Part model, mm, in its own coordinate system. Face numbers are marked on the shaded views. Give positions to 0.01 mm unless a question says otherwise; leave off trailing zeros. Order: outer loops, then holes, each group sorted by start corner. A loop starts at its lowest first (then second) coordinate and runs counter-clockwise, first axis right, second up. Notation, with made-up numbers: M 3,64 L 24,64 A21 ccw 24,76 Z; hole C 11,55 d2. An arc over 180 degrees is marked long. Return JSON: item names as keys, results as strings.
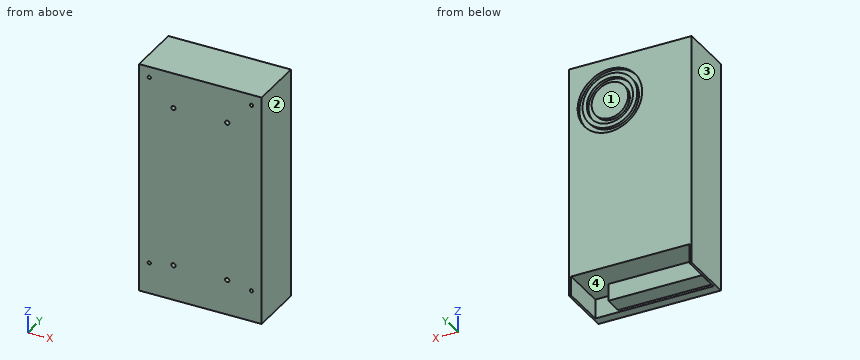
from build123d import *

# Parameters (mm, degrees)
SKETCH_2_W          = 114
SKETCH_2_H          = 216
EXTRUDE_2_DEPTH     = 51
SKETCH_3_R          = 1.5
SKETCH_3_R_2        = 2
CUT_EXTRUDE_1_DEPTH = 10
SKETCH_4_W          = 110
SKETCH_4_H          = 18
CUT_EXTRUDE_2_DEPTH = 42
SKETCH_5_W          = 87
SKETCH_5_H          = 16
EXTRUDE_3_DEPTH     = 17
SKETCH_6_R          = 30
SKETCH_6_R_2        = 25.436388115
CUT_EXTRUDE_4_DEPTH = 3
SKETCH_7_R          = 21.493717547
SKETCH_7_R_2        = 16.968980291
CUT_EXTRUDE_5_DEPTH = 3


with BuildPart() as part:
    # Эскиз2 → Бобышка-Вытянуть2 (new body)
    with BuildSketch(Plane(origin=(0, 0, 0), x_dir=(1, 0, 0), z_dir=(0, 1, 0))):
        with Locations((45.595035846, -62.514319432)):
            Rectangle(SKETCH_2_W, SKETCH_2_H)
    extrude(amount=EXTRUDE_2_DEPTH)

    # Эскиз3 → Вырез-Вытянуть1 (cut)
    with BuildSketch(Plane.XZ):
        with Locations(Location((-1.904964154, 160.514319432, 0), (0, 0, 270))):
            Circle(SKETCH_3_R)
        with Locations(Location((93.095035846, 160.514319432, 0), (0, 0, 270))):
            Circle(SKETCH_3_R)
        with Locations(Location((-1.904964154, -16.485680568, 0), (0, 0, 270))):
            Circle(SKETCH_3_R)
        with Locations(Location((93.095035846, -16.485680568, 0), (0, 0, 270))):
            Circle(SKETCH_3_R)
        with Locations(Location((20.595035846, 137.514319432, 0), (0, 0, 270))):
            Circle(SKETCH_3_R_2)
        with Locations(Location((70.595035846, 137.514319432, 0), (0, 0, 270))):
            Circle(SKETCH_3_R_2)
        with Locations(Location((20.595035846, -12.485680568, 0), (0, 0, 270))):
            Circle(SKETCH_3_R_2)
        with Locations(Location((70.595035846, -12.485680568, 0), (0, 0, 270))):
            Circle(SKETCH_3_R_2)
    extrude(amount=-CUT_EXTRUDE_1_DEPTH, mode=Mode.SUBTRACT)

    # Эскиз4 → Вырез-Вытянуть2 (cut)
    with BuildSketch(Plane(origin=(0, 51, 0), x_dir=(1, 0, 0), z_dir=(0, 1, 0))):
        with Locations((45.595035846, 36.485680568)):
            Rectangle(SKETCH_4_W, SKETCH_4_H)
    extrude(amount=-CUT_EXTRUDE_2_DEPTH, mode=Mode.SUBTRACT)

    # Эскиз5 → Бобышка-Вытянуть3 (add)
    with BuildSketch(Plane(origin=(0, 9, 0), x_dir=(1, 0, 0), z_dir=(0, 1, 0))):
        with Locations((35.880674643, 35.485680568)):
            Rectangle(SKETCH_5_W, SKETCH_5_H)
    extrude(amount=EXTRUDE_3_DEPTH)

    # Эскиз6 → Вырез-Вытянуть4 (cut)
    with BuildSketch(Plane(origin=(0, 51, 0), x_dir=(1, 0, 0), z_dir=(0, 1, 0))):
        with Locations(Location((64.595035846, -130.514319432, 0), (0, 0, 270))):
            Circle(SKETCH_6_R)
        with Locations(Location((64.595035846, -130.514319432, 0), (0, 0, 270))):
            Circle(SKETCH_6_R_2, mode=Mode.SUBTRACT)
    extrude(amount=-CUT_EXTRUDE_4_DEPTH, mode=Mode.SUBTRACT)

    # Эскиз7 → Вырез-Вытянуть5 (cut)
    with BuildSketch(Plane(origin=(0, 51, 0), x_dir=(1, 0, 0), z_dir=(0, 1, 0))):
        with Locations(Location((64.595035846, -130.514319432, 0), (0, 0, 270))):
            Circle(SKETCH_7_R)
        with Locations(Location((64.595035846, -130.514319432, 0), (0, 0, 270))):
            Circle(SKETCH_7_R_2, mode=Mode.SUBTRACT)
    extrude(amount=-CUT_EXTRUDE_5_DEPTH, mode=Mode.SUBTRACT)


solid = part.part
Q1. Pin check, flat tips, straight feed: pin 1 (13.5 mm diameter, centred on x = 53, y = 17, fed in from -Z); pin 2 (2.5 mm diameter, centred on x = -1.9, z = 160.51, fed in from -Y); pin 3 (17.5 mm diameter, centred on x = 48.5, z = -36.5, fed in from +Y). Stop position of each tip, or through.
Established:
{"pin 1": "stops at z = -43.49", "pin 2": "stops at y = 10", "pin 3": "stops at y = 26"}
Q2. Probe line 1 along X through (y, z) = (9.5, -29.5); line 2 along X through (y, z) = (8, -16.5); line 3 along Z through (x, y) = (32, 13.5). List the from-to ranges inside material, lowest first.
Established:
{"line 1": "x = -11.4 to -9.4, -7.62 to 79.38, 100.6 to 102.6", "line 2": "x = -11.4 to -3.4, -0.41 to 91.6, 94.59 to 102.6", "line 3": "z = -43.49 to 170.51"}
Q3. Two-plate mould, pull along X, no slides. Class the marked faces 1, 2, 3 and 4: +X half, -X half, draft (parallel to the pull), parting line (faces both ways), or undercut.
Established:
{"face 1": "draft", "face 2": "+X half", "face 3": "-X half", "face 4": "undercut"}
Q4. Band-saw the part on C-C (x = 54). Give the cut face in (y, z).
Established:
{"outline": "M 0,-45.49 L 9,-45.49 L 9,-43.49 L 26,-43.49 L 26,-27.49 L 51,-27.49 L 51,102.45 L 48,102.45 L 48,107.39 L 51,107.39 L 51,111.81 L 48,111.81 L 48,117.26 L 51,117.26 L 51,143.77 L 48,143.77 L 48,149.22 L 51,149.22 L 51,153.64 L 48,153.64 L 48,158.58 L 51,158.58 L 51,170.51 L 0,170.51 Z"}
Q5. Band-saw the part on A-A (y = 31). Give the cut face in (x, z), then the cut area to 3 significant figures.
Established:
{"outline": "M -11.4,-45.49 L -9.4,-45.49 L -9.4,-27.49 L 100.6,-27.49 L 100.6,-45.49 L 102.6,-45.49 L 102.6,170.51 L -11.4,170.51 Z", "area": "22,600 mm²"}
Q6. Band-saw the part on B-B (x = 10.5). Give the cut face in (y, z), then the cut area to 3 significant figures.
Established:
{"outline": "M 0,-45.49 L 9,-45.49 L 9,-43.49 L 26,-43.49 L 26,-27.49 L 51,-27.49 L 51,170.51 L 0,170.51 Z", "area": "10,500 mm²"}
